Can you work these out from the model? Positions are in its coordinate system, mm. Face numbers are marked on the shaded views. A direction names the side the tool comes from. Coordinates: 2 decimals unless noted, no trailing zeros. Order: outer loops, then holes, each group sorted by start corner. A loop starts at its lowest first (then second) coordinate and runs counter-clockwise, first axis right, second up.
```python
from build123d import *

# Parameters (mm, degrees)
F1_DEPTH     = 12
F2_START     = 4
F0_R         = 1.5
F2_DEPTH     = 4
F3_T1_DEPTH  = 58.5
F3_T3_DEPTH  = 87
F3_T5_DEPTH  = 68.5
F3_T10_ANGLE = 359.64
F3_S11_R     = 5
F3_T12_DEPTH = 7
F3_T16_ANGLE = 359.64
F3_S17_R     = 5
F3_T18_DEPTH = 7
F3_T22_ANGLE = 359.64
F3_S23_R     = 5
F3_T24_DEPTH = 7
F3_T28_ANGLE = 359.64
F3_S29_R     = 5
F3_T30_DEPTH = 7


# Not quite as in the source:
# - a fillet or chamfer that OpenCascade refuses, or shapes differently, is made with other operations: its cross-section is extruded or revolved along the edge and cut away or added


with BuildPart() as f1:
    # F0 (on Right) → F1 (new body)
    with BuildSketch(Plane.YZ):
        with BuildLine():
            Line((-6.5, -6.5), (-6.5, 0))
            Line((-6.5, 0), (-6.5, 6.5))
            Line((-6.5, 6.5), (-15, 6.5))
            Line((-15, 6.5), (-51.4245796132, 0))
            ThreePointArc((-51.4245796132, 0), (-53.3271394273, -3.8230863787), (-50, -6.5))
            Line((-50, -6.5), (-6.5, -6.5))
        make_face()
    extrude(amount=F1_DEPTH)

    # F0 (on Right) → F2 (join)
    with BuildSketch(Plane.YZ.offset(F2_START)):
        with BuildLine():
            ThreePointArc((0, -6.5), (4.5961940777, -4.5961940777), (6.5, 0))
            ThreePointArc((6.5, 0), (4.5961940777, 4.5961940777), (0, 6.5))
            ThreePointArc((0, 6.5), (-4.5961940777, 4.5961940777), (-6.5, 0))
            ThreePointArc((-6.5, 0), (-4.5961940777, -4.5961940777), (0, -6.5))
        make_face()
        Circle(F0_R, mode=Mode.SUBTRACT)
        with BuildLine():
            ThreePointArc((-6.5, 0), (-4.5961940777, 4.5961940777), (0, 6.5))
            Line((0, 6.5), (-6.5, 6.5))
            Line((-6.5, 6.5), (-6.5, 0))
        make_face()
        with BuildLine():
            Line((-6.5, -6.5), (0, -6.5))
            ThreePointArc((0, -6.5), (-4.5961940777, -4.5961940777), (-6.5, 0))
            Line((-6.5, 0), (-6.5, -6.5))
        make_face()
    extrude(amount=F2_DEPTH)

    # F3: fillet of radius 5 on 6 edges, made by hand

    # F3_s2 → F3_t1 (cut)
    with BuildSketch(Plane.XZ.offset(-6)):
        with BuildLine():
            ThreePointArc((12, 1.5), (10.5355339059, 5.0355339059), (7, 6.5))
            Line((7, 6.5), (12, 6.5))
            Line((12, 6.5), (12, 1.5))
        make_face()
        with BuildLine():
            ThreePointArc((0, 1.5), (1.4644660941, 5.0355339059), (5, 6.5))
            Line((5, 6.5), (0, 6.5))
            Line((0, 6.5), (0, 1.5))
        make_face()
    extrude(amount=F3_T1_DEPTH, mode=Mode.SUBTRACT)

    # F3_s4 → F3_t3 (cut)
    with BuildSketch(Plane(origin=(0, 23.5038661081, 4.1942866966), x_dir=(1, 0, 0), z_dir=(0, -0.9844480977, -0.1756756757))):
        with BuildLine():
            ThreePointArc((12, 4.0340477699), (10.5355339059, 7.5695816758), (7, 9.0340477699))
            Line((7, 9.0340477699), (12, 9.0340477699))
            Line((12, 9.0340477699), (12, 4.0340477699))
        make_face()
        with BuildLine():
            ThreePointArc((0, 4.0340477699), (1.4644660941, 7.5695816758), (5, 9.0340477699))
            Line((5, 9.0340477699), (0, 9.0340477699))
            Line((0, 9.0340477699), (0, 4.0340477699))
        make_face()
    extrude(amount=F3_T3_DEPTH, mode=Mode.SUBTRACT)

    # F3_s6 → F3_t5 (cut)
    with BuildSketch(Plane.XZ.offset(-6)):
        with BuildLine():
            ThreePointArc((5, -6.5), (1.4644660941, -5.0355339059), (0, -1.5))
            Line((0, -1.5), (0, -6.5))
            Line((0, -6.5), (5, -6.5))
        make_face()
        with BuildLine():
            ThreePointArc((7, -6.5), (10.5355339059, -5.0355339059), (12, -1.5))
            Line((12, -1.5), (12, -6.5))
            Line((12, -6.5), (7, -6.5))
        make_face()
    extrude(amount=F3_T5_DEPTH, mode=Mode.SUBTRACT)


with BuildPart() as f3_tool8:
    # F3_s9 → F3_t10 (revolve)
    with BuildSketch(Plane(origin=(0, -50.0174650791, -0.3142731374), x_dir=(1, 0, 0), z_dir=(0, -0.9999802609, -0.006283144))):
        with BuildLine():
            ThreePointArc((7, -6.185781731), (9.9180943161, -5.2459203447), (11.7391469644, -2.779671956))
            Line((11.7391469644, -2.779671956), (12, -2.779671956))
            Line((12, -2.779671956), (12, -6.185781731))
            Line((12, -6.185781731), (7, -6.185781731))
        make_face()
    revolve(axis=Axis((12, -50, -3.093890225), (1, 0, 0)), revolution_arc=F3_T10_ANGLE)

    # F3_s11 → F3_t12 (cut, symmetric)
    with BuildSketch(Plane(origin=(0, -49.0255152632, -8.7486486486), x_dir=(1, 0, 0), z_dir=(0, 0.9844480977, 0.1756756757))):
        with Locations((7, -4.0340477699)):
            Circle(F3_S11_R)
    extrude(amount=F3_T12_DEPTH, both=True, mode=Mode.SUBTRACT)


with BuildPart() as f1_1:
    add(f1.part)

    # F3_t7: cut F3_tool8
    add(f3_tool8.part, mode=Mode.SUBTRACT)


with BuildPart() as f3_tool14:
    # F3_s15 → F3_t16 (revolve)
    with BuildSketch(Plane(origin=(0, -50.0174650791, -0.3142731374), x_dir=(1, 0, 0), z_dir=(0, -0.9999802609, -0.006283144))):
        with BuildLine():
            ThreePointArc((7, -6.185781731), (9.9180943161, -5.2459203447), (11.7391469644, -2.779671956))
            Line((11.7391469644, -2.779671956), (12, -2.779671956))
            Line((12, -2.779671956), (12, -6.185781731))
            Line((12, -6.185781731), (7, -6.185781731))
        make_face()
    revolve(axis=Axis((12, -50, -3.093890225), (1, 0, 0)), revolution_arc=F3_T16_ANGLE)

    # F3_s17 → F3_t18 (cut, symmetric)
    with BuildSketch(Plane.XZ.offset(50)):
        with Locations((7, -1.5)):
            Circle(F3_S17_R)
    extrude(amount=F3_T18_DEPTH, both=True, mode=Mode.SUBTRACT)


with BuildPart() as f1_2:
    add(f1_1.part)

    # F3_t13: cut F3_tool14
    add(f3_tool14.part, mode=Mode.SUBTRACT)


with BuildPart() as f3_tool20:
    # F3_s21 → F3_t22 (revolve)
    with BuildSketch(Plane(origin=(0, -50.0174650791, -0.3142731374), x_dir=(1, 0, 0), z_dir=(0, -0.9999802609, -0.006283144))):
        with BuildLine():
            ThreePointArc((5, -6.185781731), (2.0819056839, -5.2459203447), (0.2608530356, -2.779671956))
            Line((0.2608530356, -2.779671956), (0, -2.779671956))
            Line((0, -2.779671956), (0, -6.185781731))
            Line((0, -6.185781731), (5, -6.185781731))
        make_face()
    revolve(axis=Axis((0, -50, -3.093890225), (1, 0, 0)), revolution_arc=F3_T22_ANGLE)

    # F3_s23 → F3_t24 (cut, symmetric)
    with BuildSketch(Plane(origin=(0, -49.0255152632, -8.7486486486), x_dir=(1, 0, 0), z_dir=(0, 0.9844480977, 0.1756756757))):
        with Locations((5, -4.0340477699)):
            Circle(F3_S23_R)
    extrude(amount=F3_T24_DEPTH, both=True, mode=Mode.SUBTRACT)


with BuildPart() as f1_3:
    add(f1_2.part)

    # F3_t19: cut F3_tool20
    add(f3_tool20.part, mode=Mode.SUBTRACT)


with BuildPart() as f3_tool26:
    # F3_s27 → F3_t28 (revolve)
    with BuildSketch(Plane(origin=(0, -50.0174650791, -0.3142731374), x_dir=(1, 0, 0), z_dir=(0, -0.9999802609, -0.006283144))):
        with BuildLine():
            ThreePointArc((5, -6.185781731), (2.0819056839, -5.2459203447), (0.2608530356, -2.779671956))
            Line((0.2608530356, -2.779671956), (0, -2.779671956))
            Line((0, -2.779671956), (0, -6.185781731))
            Line((0, -6.185781731), (5, -6.185781731))
        make_face()
    revolve(axis=Axis((0, -50, -3.093890225), (1, 0, 0)), revolution_arc=F3_T28_ANGLE)

    # F3_s29 → F3_t30 (cut, symmetric)
    with BuildSketch(Plane.XZ.offset(50)):
        with Locations((5, -1.5)):
            Circle(F3_S29_R)
    extrude(amount=F3_T30_DEPTH, both=True, mode=Mode.SUBTRACT)


with BuildPart() as f1_4:
    add(f1_3.part)

    # F3_t25: cut F3_tool26
    add(f3_tool26.part, mode=Mode.SUBTRACT)


solid = f1_4.part
```
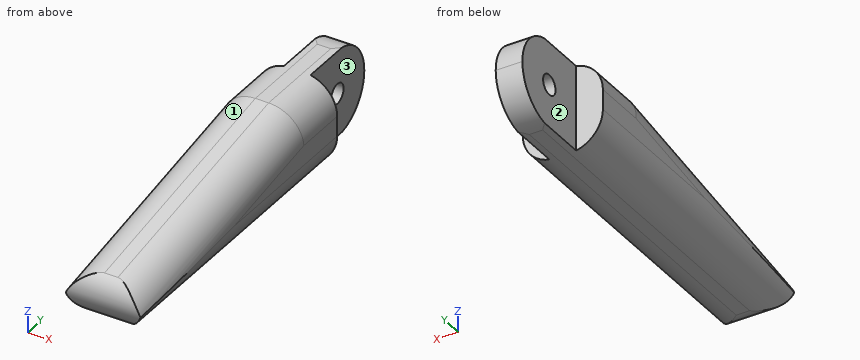
1. Imagine slicing it at A-A on y = -10.5. Please give me the cut outline in (x, z), then the cut area to 3 significant figures.
Completed:
outline: (0, -1.5) arc R5 ccw to (5, -6.5) - (7, -6.5) arc R5 ccw to (12, -1.5) - (12, 1.5) arc R5 ccw to (7, 6.5) - (5, 6.5) arc R5 ccw to (0, 1.5) - close
area: 135 mm2
2. I'm going to push flat-ended pins straight in: pin 1 (6 mm diameter, centred on x = 3.5, z = -3.5, fed in from -Y); pin 2 (3 mm diameter, centred on x = 10, y = -25, fed in from -Z); pin 3 (1.2 mm diameter, centred on x = 9.5, z = 3, fed in from +Y). Where does each tip first touch, or does it pass through?
Completed:
pin 1: stops at y = -53.41
pin 2: stops at z = -6.27
pin 3: stops at y = -6.5
3. Please list where these lines run through material, in increasing order: probe 1 along Z at (x, y) = (5.25, 0); probe 2 along X at (y, z) = (-25, -0.25); probe 3 along X at (y, z) = (-3.5, 0.75).
Completed:
probe 1: z = -6.5 to -1.5, 1.5 to 6.5
probe 2: x = 0 to 12
probe 3: x = 4 to 8
4. Imagine slicing it at B-B on z = -5.5. Please give me the cut outline in (x, y), then the cut area to 3 significant figures.
Completed:
outline: (2, -52.41) - (10, -52.41) - (10, -6.5) - (8, -6.5) - (8, 3.46) - (4, 3.46) - (4, -6.5) - (2, -6.5) - close
area: 407 mm2
5. Imagine slicing it at C-C on x = 10.25. Please give me the cut outline in (y, z), then the cut area to 3 significant figures.
Completed:
outline: (-53.01, -1.5) arc R3.41 ccw to (-52.6, -5.3) - (-6.5, -5.3) - (-6.5, 5.3) - (-14.89, 5.3) - close
area: 364 mm2
6. Imagine slicing it at D-D on x = 2. Please give me the cut outline in (y, z).
Completed:
outline: (-52.88, -1.28) arc R3.41 ccw to (-52.41, -5.5) - (-6.5, -5.5) - (-6.5, 5.5) - (-14.91, 5.5) - close
7. On a 3-axis mill with a long thin cutter (end or side, diameter ignored), from which of +Z, -Z, +X, -X, +Y, -Y can I reach the whole of each face in a straight line? I mean the marked faces 1, 2 and 3. Say none if no direction works.
Completed:
face 1: +Z, -X, -Y
face 2: +Z, -Z, -X, +Y
face 3: +Z, -Z, +X, +Y
